Answer from the drawing. Dimensions are ordinates in mm from the lowest x, y and z of the part. A direction names the side the tool comes from. Round coordinates to 2 decimals unless told otherwise and drop trailing zeros. Order: outer loops, then holes, each group sorted by start corner. A loop starts at its lowest first (then second) coordinate and runs counter-clockwise, first axis right, second up. Notation, with made-up numbers: M 89.5,22 L 147.5,22 A25 cw 147.5,41 Z; hole C 88,33.25 d11. An arc over 180 degrees is marked long. Write item = value, one per line. Start each with the question number.
(1) Straight lines are drawn through the part: probe 1 along X at (y, z) = (17, 12.5); probe 2 along Y at (x, z) = (25, 5.5); probe 3 along Y at (x, z) = (24, 11.25). For each, find the intervals that lie inside material, in ascending order. Write a range as from..to.
(2) Which of the six approach directions +Z, -Z, +X, -X, +Y, -Y give full straight-line access (tool end or side, diameter ignored) to the marked faces 1, 2 and 3?
(3) A cutting plane is placed at D-D, the plane z = 18. Determine the outline of the cut face in (x, y), and give its area (3 significant figures).
(4) A cutting plane is placed at C-C, the plane x = 25. Determine the outline of the cut face in (y, z).
(5) A cutting plane is placed at A-A, the plane y = 10. Determine the outline of the cut face in (x, z).
(6) Each of these flat-tipped pins is pushed along its axis until it touches: pin 1 (4 mm diameter, centred on y = 16.5, z = 5.5, fed in from +X); pin 2 (8 mm diameter, centred on x = 11, y = 3.5, fed in from +Z); pin 3 (3 mm diameter, centred on x = 36.5, z = 15, fed in from +Y); pin 4 (6 mm diameter, centred on x = 25, y = 10, fed in from +Z). Where does it stop, or does it pass through?
(7) A cutting plane is placed at B-B, the plane z = 10. Determine the outline of the cut face in (x, y), and give its area (3 significant figures).
(8) For a pull along X with two mould halves and no side action, classify the marked faces 4, 5 and 6 as released by +X, released by -X, zero draft, split by the parting line, or undercut.
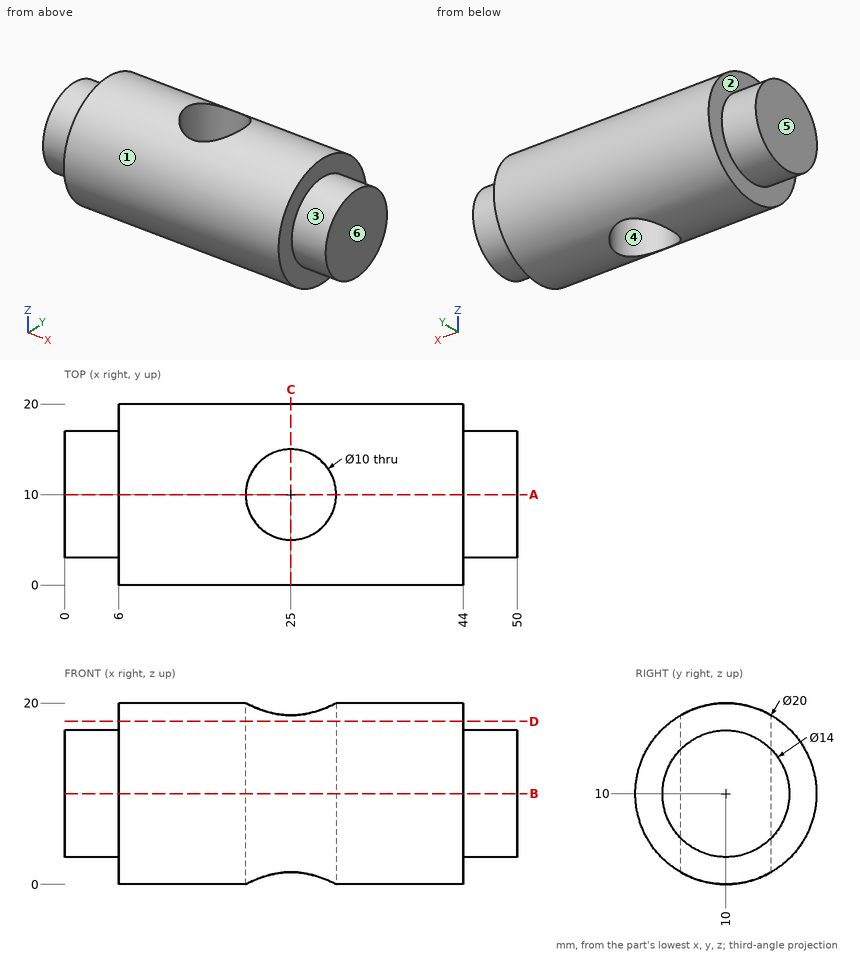
Reported:
q1.probe_1 = 6..44
q1.probe_2 = 1.07..5, 15..18.93
q1.probe_3 = 0.08..5.1, 14.9..19.92
q2.face_1 = +X, -X
q2.face_2 = -X
q2.face_3 = +X
q3.outline = M 6,4 L 44,4 L 44,16 L 6,16 Z; hole C 25,10 d10
q3.area = 377 mm²
q4.outline = M 5,1.34 L 5,18.66 A10 ccw Z; M 15,1.34 A10 ccw 15,18.66 Z
q5.outline = M 0,3 L 6,3 L 6,0 L 20,0 L 20,20 L 6,20 L 6,17 L 0,17 Z; M 30,0 L 44,0 L 44,3 L 50,3 L 50,17 L 44,17 L 44,20 L 30,20 Z
q6.pin_1 = 50
q6.pin_2 = 19.68
q6.pin_3 = 19.37
q6.pin_4 = through
q7.outline = M 0,3 L 6,3 L 6,0 L 44,0 L 44,3 L 50,3 L 50,17 L 44,17 L 44,20 L 6,20 L 6,17 L 0,17 Z; hole C 25,10 d10
q7.area = 849 mm²
q8.face_4 = undercut
q8.face_5 = released by -X
q8.face_6 = released by +X
